```python
from build123d import *

# Parameters (mm, degrees)
SKIZZE7_R                            = 5
AUFSATZ_LINEAR_AUSTRAGEN4_DEPTH      = 10
SCHNITT_LINEAR_AUSTRAGEN2_DEPTH      = 13.247448714
SCHNITT_LINEAR_AUSTRAGEN2_DEPTH_BACK = 13.247448714
SKIZZE8_W                            = 10
SKIZZE8_H                            = 6
SCHNITT_LINEAR_AUSTRAGEN3_DEPTH      = 13.247448714
SCHNITT_LINEAR_AUSTRAGEN3_DEPTH_BACK = 13.247448714
SKIZZE5_R                            = 1
SKIZZE5_W                            = 10
SKIZZE5_H                            = 3
VERRUNDUNG1_R                        = 2


with BuildPart() as part:
    # Skizze7 → Aufsatz-Linear austragen4 (new, symmetric)
    with BuildSketch(Plane(origin=(0, 0, 0), x_dir=(0, 0, -1), z_dir=(1, 0, 0))):
        Circle(SKIZZE7_R)
    extrude(amount=AUFSATZ_LINEAR_AUSTRAGEN4_DEPTH, both=True)

    # Skizze8 → Schnitt-Linear austragen2 (cut, two sides: drawn at the far end of the back side and taken through both)
    with BuildSketch(Plane.XY.offset(-SCHNITT_LINEAR_AUSTRAGEN2_DEPTH_BACK)):
        with Locations((5, 0)):
            Rectangle(SKIZZE8_W, SKIZZE8_H)
    extrude(amount=SCHNITT_LINEAR_AUSTRAGEN2_DEPTH + SCHNITT_LINEAR_AUSTRAGEN2_DEPTH_BACK, mode=Mode.SUBTRACT)

    # Skizze5 → Schnitt-Linear austragen3 (cut, two sides: drawn at the far end of the back side and taken through both)
    with BuildSketch(Plane(origin=(0, 0, 0), x_dir=(1, 0, 0), z_dir=(0, 1, 0)).offset(-SCHNITT_LINEAR_AUSTRAGEN3_DEPTH_BACK)):
        with Locations(Location((6, 0, 0), (0, 0, 270))):
            Circle(SKIZZE5_R)
        with Locations((5, 3.5)):
            Rectangle(SKIZZE5_W, SKIZZE5_H)
        with Locations((5, -3.5)):
            Rectangle(SKIZZE5_W, SKIZZE5_H)
    extrude(amount=SCHNITT_LINEAR_AUSTRAGEN3_DEPTH + SCHNITT_LINEAR_AUSTRAGEN3_DEPTH_BACK, mode=Mode.SUBTRACT)

    # Verrundung1
    verrundung1_edges = [part.edges().sort_by_distance(p)[0] for p in [
        (10, -3.791287847, -2),
        (10, -3.791287847, 2),
        (10, 3.791287847, -2),
        (10, 3.791287847, 2),
    ]]
    fillet(verrundung1_edges, radius=VERRUNDUNG1_R - 0.0001)  # a hair under: the kernel refuses the full size


solid = part.part
```
Can you work these out from the model? Positions are in its coordinate system, mm. A direction names the side the tool comes from. Coordinates: 2 decimals unless noted, no trailing zeros. Write each loop counter-clockwise with the first axis right and the second up, starting at its lowest first coordinate (ties: lowest second). Pieces come first, ordered by that corner, then holes. Notation, with made-up numbers: M 18,33 L 40,33 A21 cw 40,69 Z; hole C 51,34 d2. An arc over 180 degrees is marked long. Answer as CSV lines item,"result".
Item 1: Imagine slicing it at D-D on y = 0. List the corners of the cut face in (x, z) for me.
Geometry results:
outline,"M -10,-5 L 0,-5 L 0,5 L -10,5 Z"
Item 2: Imagine slicing it at C-C on z = -0.5. List the corners of the cut face in (x, y) for me.
Geometry results:
outline,"M -10,-4.97 L 5.13,-4.97 L 5.13,-3 L 0,-3 L 0,3 L 5.13,3 L 5.13,4.97 L -10,4.97 Z; M 6.87,-4.97 L 9.94,-4.97 L 9.94,-3 L 6.87,-3 Z; M 6.87,3 L 9.94,3 L 9.94,4.97 L 6.87,4.97 Z"
Item 3: We'd pull the mould along Z, two halves only. Please class faces 4 (the flat face through (4, 4, -2)), 5 (the cylindrical face through (7, 4, 0)), 6 (the cylindrical face through (9.4, -3.99, 1.43)): +Z half, -Z half, draft (parallel to the pull), parting line (faces both ways), or undercut.
Geometry results:
face 4,"-Z half"
face 5,"undercut"
face 6,"+Z half"
Item 4: Please list where these lines run through material, in increasing order: line 1 along Z through (x, y) = (6, 4.05); line 2 along X through (y, z) = (4.6, 0); line 3 along X through (y, z) = (3, 3.25).
Geometry results:
line 1,"z = -2 to -1, 1 to 2"
line 2,"x = -10 to 5, 7 to 10"
line 3,"x = -10 to 0"
Item 5: On a 3-axis mill with a long thin cutter (end or side, diameter ignored), from which of +Z, -Z, +X, -X, +Y, -Y can I reach the whole of each face in a straight line? I mean faces 1 (the flat face through (4, -4, -2)), 2 (the flat face through (4, -4, 2)), 3 (the flat face through (4.9, -3, 0.4)). Say none if no direction works.
Geometry results:
face 1,"-Z, +X, +Y, -Y"
face 2,"+Z, +X, +Y, -Y"
face 3,"+Z, -Z, +X"
Item 6: I'm going to push flat-ended pins straight in: P1, Ø0.5, axis at x = 5.5, y = 3.5, coming from the -Z side; P2, Ø1.3, axis at x = 5, y = -3.5, coming from the +Z side; P3, Ø1.5, axis at y = 2, z = 0.5, coming from the +X side. Where does each tip first touch, or does it pass through?
Geometry results:
P1,"stops at z = -2"
P2,"stops at z = 2"
P3,"stops at x = 0"
Item 7: Imagine slicing it at A-A on x = 7.25. List the corners of the cut face in (y, z) for me, plus the area to 3 significant figures.
Geometry results:
outline,"M -4.58,-2 L -3,-2 L -3,2 L -4.58,2 A5 ccw Z; M 3,-2 L 4.58,-2 A5 ccw 4.58,2 L 3,2 Z"
area,"14.9 mm2"
